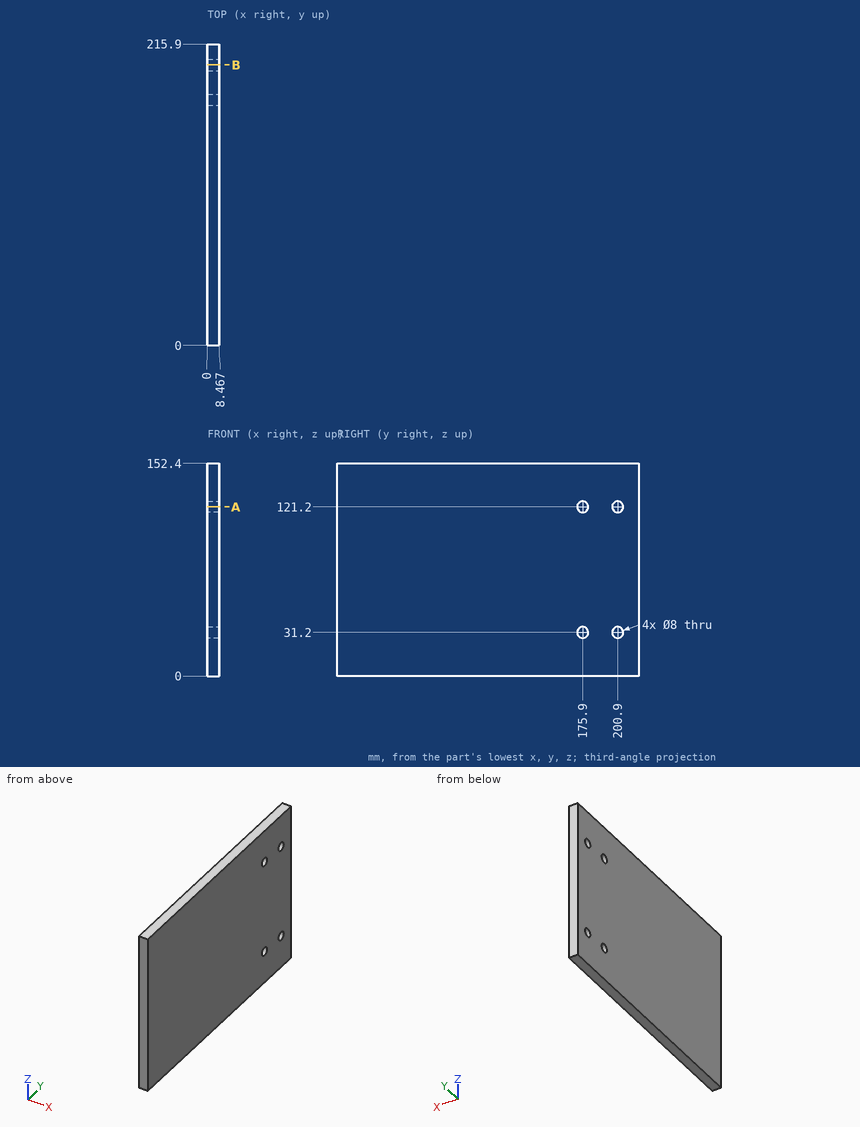
Geometry check sheet. Reference: drawing and pictorial views, mm from the part's lowest x, y, z. Round coordinates to 2 decimals unless told otherwise and drop trailing zeros. Loops run counter-clockwise (first coordinate to the right, second up) from the corner with the lowest first, then second, coordinate; pieces in that order, holes last. Notation, with made-up numbers: (43, 16) - (74, 16) arc R9 ccw to (74, 21) - close; hole circle Ø11 at (57.25, -28). An arc over 180 degrees is marked (long way). Use a Markdown table: item, result.
Q1. Go/stop test with a flat-tipped pin: P1, Ø4, axis at x = 1, z = 127, coming from the -Y side. Record where the tip stops, or that it passes through.
Solutions:
| item | result |
|---|---|
| P1 | stops at y = 0 |
Q2. Cross-section at B-B on y = 200.9. Record the cut outline in (x, z), plus the area to 4 significant figures.
Solutions:
| item | result |
|---|---|
| outline | (0, 0) - (8.47, 0) - (8.47, 27.2) - (0, 27.2) - close; (0, 35.2) - (8.47, 35.2) - (8.47, 117.2) - (0, 117.2) - close; (0, 125.2) - (8.47, 125.2) - (8.47, 152.4) - (0, 152.4) - close |
| area | 1,155 mm2 |
Q3. Cross-section at A-A on z = 121.2. Record the cut outline in (x, y), plus the area to 3 significant figures.
Solutions:
| item | result |
|---|---|
| outline | (0, 0) - (8.47, 0) - (8.47, 171.9) - (0, 171.9) - close; (0, 179.9) - (8.47, 179.9) - (8.47, 196.9) - (0, 196.9) - close; (0, 204.9) - (8.47, 204.9) - (8.47, 215.9) - (0, 215.9) - close |
| area | 1,690 mm2 |
Q4. Material ranges on line 1 (Y direction, x = 6, z = 31.2); line 2 (Y direction, x = 6.5, z = 33.5); line 3 (Z direction, x = 7.5, y = 173.5), recorded low to high.
Solutions:
| item | result |
|---|---|
| line 1 | y = 0 to 171.9, 179.9 to 196.9, 204.9 to 215.9 |
| line 2 | y = 0 to 172.63, 179.17 to 197.63, 204.17 to 215.9 |
| line 3 | z = 0 to 28, 34.4 to 118, 124.4 to 152.4 |
